Design review of the part shown in the three views and the two pictorial views. Dimensions are in mm from the part's minimum x, y and z. A direction names the side the tool comes from. Coordinates: 2 decimals unless noted, no trailing zeros. Write each loop counter-clockwise with the first axis right and the second up, starting at its lowest first coordinate (ties: lowest second). Pieces come first, ordered by that corner, then holes. Notation, with made-up numbers: M 87.5,67 L 95.5,67 A27 ccw 95.5,101 Z; hole C 36.25,40.25 d6. An arc over 180 degrees is marked long. Answer as a JSON object with one key per item and string values.
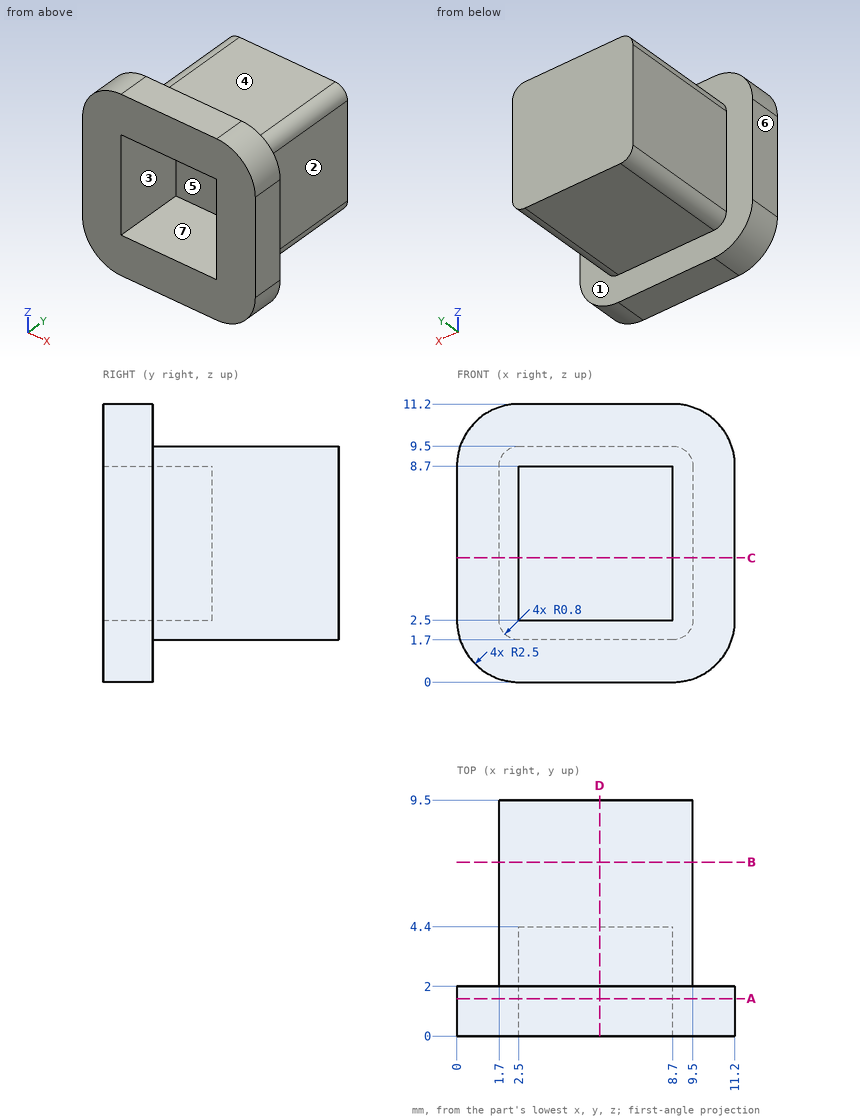
(1) Add section B-B on y = 7. Give the boundary of the cut face in (x, z), and give its area (3 significant figures).
Results list:
{"outline": "M 1.7,2.5 A0.8 ccw 2.5,1.7 L 8.7,1.7 A0.8 ccw 9.5,2.5 L 9.5,8.7 A0.8 ccw 8.7,9.5 L 2.5,9.5 A0.8 ccw 1.7,8.7 Z", "area": "60.3 mm²"}
(2) Draft analysis for pull direction X (two halves, no side actions). For the marked faces 4, 5, 6 and 7, state which applies: released by +X, released by -X, zero draft, split by the parting line, or undercut.
Results list:
{"face 4": "zero draft", "face 5": "undercut", "face 6": "released by -X", "face 7": "undercut"}
(3) Add section C-C on z = 5. Give the boundary of the cut face in (x, y), and give its area (3 significant figures).
Results list:
{"outline": "M 0,0 L 2.5,0 L 2.5,4.4 L 8.7,4.4 L 8.7,0 L 11.2,0 L 11.2,2 L 9.5,2 L 9.5,9.5 L 1.7,9.5 L 1.7,2 L 0,2 Z", "area": "53.6 mm²"}
(4) For the marked faces 1, 2 and 3, list the 3-axis set-ups (+Z, -Z, +X, -X, +Y, -Y) from which the entire face can be reached by the end or side of a thin tool; tool diameter is ignored.
Results list:
{"face 1": "+Y", "face 2": "+Z, -Z, +X, +Y", "face 3": "-Y"}
(5) For pin 1 Ø1 at (y, z) = (2, 9.5) entering from +X; pin 2 Ø3 at (y, z) = (5, 6) entering from +X; pin 3 Ø3 at (x, y) = (4, 5.5) entering from +Z, all flat-tipped, find the tip position at first contact; note any pin that passes through.
Results list:
{"pin 1": "x = 11.18", "pin 2": "x = 9.5", "pin 3": "z = 9.5"}
(6) Add section A-A on y = 1.5. Give the boundary of the cut face in (x, z), and give its area (3 significant figures).
Results list:
{"outline": "M 0,2.5 A2.5 ccw 2.5,0 L 8.7,0 A2.5 ccw 11.2,2.5 L 11.2,8.7 A2.5 ccw 8.7,11.2 L 2.5,11.2 A2.5 ccw 0,8.7 Z; hole M 2.5,2.5 L 8.7,2.5 L 8.7,8.7 L 2.5,8.7 Z", "area": "81.6 mm²"}
(7) Add section D-D on x = 5.75. Give the boundary of the cut face in (y, z).
Results list:
{"outline": "M 0,0 L 2,0 L 2,1.7 L 9.5,1.7 L 9.5,9.5 L 2,9.5 L 2,11.2 L 0,11.2 L 0,8.7 L 4.4,8.7 L 4.4,2.5 L 0,2.5 Z"}
(8) Wall thickness on line 1 along X through (y, z) = (2.5, 7.5); line 2 along X through (y, z) = (8.25, 6.5): over which ranges is each line inside the solid? List them lowest first. Write a range as from..to.
Results list:
{"line 1": "1.7..2.5, 8.7..9.5", "line 2": "1.7..9.5"}
